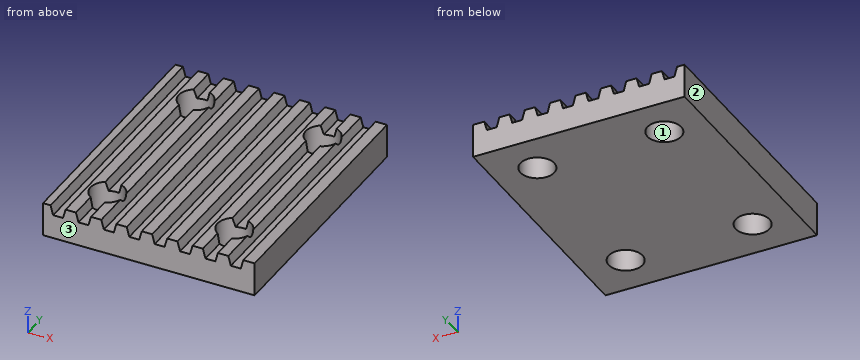
Autodesk Fusion 360 part; units mm, degrees
sketch "Sketch1" plane through (0, 0, 0) normal (0, 0, 1) x (1, 0, 0)
  line L0 (0, 0) -> (25, 0)
  line L1 (25, 0) -> (25, 30)
  line L2 (25, 30) -> (0, 30)
  line L3 (0, 30) -> (0, 0)
  dimension "d1" = 25
  dimension "d2" = 30
extrude "Extrude1" add sketch "Sketch1" along normal blind 4
sketch "Sketch2" plane through (0, 0, 0) normal (0, -1, 0) x (1, 0, 0)
  line L0 (0, 0) -> (25, 0)
  line L1 (25, 0) -> (25, 4)
  line L2 (25, 4) -> (0, 4)
  line L3 (0, 4) -> (0, 0)
  line L4 (25, 2.86) -> (0, 2.86)
  line L5 (0.89, 4) -> (1.1955, 2.86)
  line L6 (2.3645, 2.86) -> (2.67, 4)
  line L7 (3.89, 4) -> (4.1955, 2.86)
  line L8 (5.3645, 2.86) -> (5.67, 4)
  line L9 (6.89, 4) -> (7.1955, 2.86)
  line L10 (8.3645, 2.86) -> (8.67, 4)
  line L11 (9.89, 4) -> (10.1955, 2.86)
  line L12 (11.3645, 2.86) -> (11.67, 4)
  line L13 (12.89, 4) -> (13.1955, 2.86)
  line L14 (14.3645, 2.86) -> (14.67, 4)
  line L15 (15.89, 4) -> (16.1955, 2.86)
  line L16 (17.3645, 2.86) -> (17.67, 4)
  line L17 (18.89, 4) -> (19.1955, 2.86)
  line L18 (20.3645, 2.86) -> (20.67, 4)
  line L19 (21.89, 4) -> (22.1955, 2.86)
  line L20 (23.3645, 2.86) -> (23.67, 4)
  dimension "d5" = 1.14
  dimension "d7" = 1.78
  dimension "d8" = 0.89
  dimension "d11" = 3
  dimension "d12" = 0
  dimension "d15" = 30
extrude "Extrude2" cut sketch "Sketch2" against normal up to surface (30 mm away) contours L2 L4 L5 L6 | L2 L4 L19 L20 | L2 L4 L7 L8 | L2 L4 L17 L18 | L2 L4 L9 L10 | L2 L4 L15 L16 | L2 L4 L11 L12 | L2 L4 L13 L14
sketch "Sketch3" plane through (0, 0, 0) normal (0, 0, -1) x (1, 0, 0)
  line L0 (0, 0) -> (0, -30)
  line L1 (0, -30) -> (25, -30)
  line L2 (25, -30) -> (25, 0)
  line L3 (25, 0) -> (0, 0)
  line L4 (20, -25) -> (5, -25) construction
  line L5 (5, -25) -> (5, -5) construction
  line L6 (5, -5) -> (20, -5) construction
  line L7 (20, -5) -> (20, -25) construction
  circle A0 centre (20, -25) radius 2
  circle A1 centre (5, -25) radius 2
  circle A2 centre (20, -5) radius 2
  circle A3 centre (5, -5) radius 2
  point P0 (12.5, -25)
  point P1 (5, -15)
  point P2 (0, -15)
  point P3 (12.5, -30)
  dimension "d16" = 15
  dimension "d17" = 20
  dimension "d18" = 4
  dimension "d19" = 4
extrude "Extrude3" cut sketch "Sketch3" against normal through all contours A0 | A1 | A2 | A3
equation "d8 = ( 1.78 / 2 ) * 1 mm"
Can you work these out from the model? Positions are in its coordinate system, mm. Face numbers are marked on the shaded views. Coordinates: 2 decimals unless noted, no trailing zeros. Order: outer loops, then holes, each group sorted by start corner. A loop starts at its lowest first (then second) coordinate and runs counter-clockwise, first axis right, second up. Notation, with made-up numbers: (49, -31) -> (56, -31) arc R19 ccw to (56, -24) -> close; hole circle Ø9 at (16.5, 55). An arc over 180 degrees is marked (long way). Write each question's results on one line, items separated by ' | '.
Item 1: I want a section at D-D, the plane x = 8. Write out the boundary of the cut face in (y, z), then the cut area to 3 significant figures.
Results are:
outline: (0, 0) -> (30, 0) -> (30, 2.86) -> (0, 2.86) -> close | area: 85.8 mm²
Item 2: I want a section at C-C, the plane y = 5. Count the separate pieces of the cut face and the enclosed holes in it, then the cut area to 3 significant figures.
Results are:
separate pieces: 3 | enclosed holes: 0 | area: 58.0 mm²
Item 3: I'm going to push flat-ended pins straight in: pin 1 Ø3 at (x, y) = (11.5, 14.5) entering from -Z; pin 2 Ø3.5 at (x, y) = (5, 25) entering from +Z; pin 3 Ø0.6 at (x, y) = (8, 10.5) entering from +Z. Where does each tip first touch, or does it pass through?
Results are:
pin 1: z = 0 | pin 2: through | pin 3: z = 2.86
Item 4: I want a section at A-A, the plane x = 20. Write out the boundary of the cut face in (y, z), then the cut area to 3 significant figures.
Results are:
outline: (0, 0) -> (3, 0) -> (3, 2.86) -> (0, 2.86) -> close; (7, 0) -> (23, 0) -> (23, 2.86) -> (7, 2.86) -> close; (27, 0) -> (30, 0) -> (30, 2.86) -> (27, 2.86) -> close | area: 62.9 mm²
Item 5: I want a section at B-B, the plane z = 1.25. Write out the boundary of the cut face in (x, y).
Results are:
outline: (0, 0) -> (25, 0) -> (25, 30) -> (0, 30) -> close; hole circle Ø4 at (5, 5); hole circle Ø4 at (5, 25); hole circle Ø4 at (20, 5); hole circle Ø4 at (20, 25)
Item 6: If I drill on line 1 along Y through (x, z) = (20, 2.2); line 2 along X through (y, z) = (5, 1.4); line 3 along X through (y, z) = (26.25, 2.5), over which ranges is the centre line in solid material (lowest first)?
Results are:
line 1: 0 to 3, 7 to 23, 27 to 30 | line 2: 0 to 3, 7 to 18, 22 to 25 | line 3: 0 to 3.44, 6.56 to 18.44, 21.56 to 25
Item 7: If we mould it in two halves opening along X, with no side actions, what happens to the marked faces 1, 2 and 3? For each: +X half, -X half, draft (parallel to the pull), parting line (faces both ways), or undercut.
Results are:
face 1: undercut | face 2: -X half | face 3: draft
